from build123d import *

# Parameters (mm, degrees)
F0_W     = 4.5
F0_H     = 2.2
F1_DEPTH = 0.6
F2_W     = 4.5
F2_H     = 2.2
F3_DEPTH = 1.6
F4_R     = 1.09999
F5_R     = 0.5
F6_DEPTH = 25


# Not quite as in the source:
# - a fillet or chamfer is up to 0.001 mm smaller than in the source, because OpenCascade refuses the exact size


with BuildPart() as f1:
    # F0 (on Top) → F1 (new body)
    with BuildSketch(Plane.XY):
        with Locations((9.75, 2.6)):
            Rectangle(F0_W, F0_H)
        with BuildLine():
            Line((7.0565025569, 1.5), (7.5, 1.5))
            Line((7.5, 1.5), (7.5, 3.7))
            Line((7.5, 3.7), (7.0565025569, 3.7))
            ThreePointArc((7.0565025569, 3.7), (6.7766250144, 3.7151076306), (6.5, 3.7602549529))
            ThreePointArc((6.5, 3.7602549529), (6.2418088438, 3.8309365837), (5.9922537502, 3.9277912239))
            Line((5.9922537502, 3.9277912239), (3.6642488067, 4.9722087761))
            ThreePointArc((3.6642488067, 4.9722087761), (4.7825497586, 4.012967286), (5.2, 2.6))
            ThreePointArc((5.2, 2.6), (4.7825497586, 1.187032714), (3.6642488067, 0.2277912239))
            Line((3.6642488067, 0.2277912239), (5.9922537502, 1.2722087761))
            ThreePointArc((5.9922537502, 1.2722087761), (6.2418088438, 1.3690634163), (6.5, 1.4397450471))
            ThreePointArc((6.5, 1.4397450471), (6.7766250144, 1.4848923694), (7.0565025569, 1.5))
        make_face()
        with BuildLine():
            ThreePointArc((2.6, 0), (3.1441769851, 0.0575855159), (3.6642488067, 0.2277912239))
            ThreePointArc((3.6642488067, 0.2277912239), (4.7825497586, 1.187032714), (5.2, 2.6))
            ThreePointArc((5.2, 2.6), (4.7825497586, 4.012967286), (3.6642488067, 4.9722087761))
            ThreePointArc((3.6642488067, 4.9722087761), (3.1441769851, 5.1424144841), (2.6, 5.2))
            Line((2.6, 5.2), (2.6, 4.2))
            ThreePointArc((2.6, 4.2), (3.7313708499, 3.7313708499), (4.2, 2.6))
            ThreePointArc((4.2, 2.6), (3.7313708499, 1.4686291501), (2.6, 1))
            Line((2.6, 1), (2.6, 0))
        make_face()
        with BuildLine():
            ThreePointArc((0, 2.6), (0.7615223689, 0.7615223689), (2.6, 0))
            Line((2.6, 0), (2.6, 1))
            ThreePointArc((2.6, 1), (1, 2.6), (2.6, 4.2))
            Line((2.6, 4.2), (2.6, 5.2))
            ThreePointArc((2.6, 5.2), (0.7615223689, 4.4384776311), (0, 2.6))
        make_face()
    extrude(amount=F1_DEPTH)

    # F2 (on face) → F3 (join)
    with BuildSketch(Plane.XY.offset(0.6)):
        with Locations((9.75, 2.6)):
            Rectangle(F2_W, F2_H)
    extrude(amount=F3_DEPTH)

    # F4 (radius 1.1 in the source; OpenCascade refuses exactly that, so slightly less here)
    f4_edges = [f1.edges().sort_by_distance(p)[0] for p in [
        (9.75, 3.7, 2.2),
        (9.75, 1.5, 2.2),
    ]]
    fillet(f4_edges, radius=F4_R)

    # F5 (on face) → F6 (cut)
    with BuildSketch(Plane.YZ.offset(12)):
        with Locations((2.6, 1.1)):
            Circle(F5_R)
    extrude(amount=-F6_DEPTH, mode=Mode.SUBTRACT)


solid = f1.part
Verification items for the finished model (mm, model axes). A direction names the side the tool comes from. Coordinates: 2 decimals unless noted, no trailing zeros. Loops run counter-clockwise (first coordinate to the right, second up) from the corner with the lowest first, then second, coordinate; pieces in that order, holes last. Notation, with made-up numbers: (78.25, -19) -> (83.25, -19) arc R24 ccw to (83.25, 8) -> close; hole circle Ø11 at (14.5, 83.25). An arc over 180 degrees is marked (long way). Answer as CSV lines item,"result".
1) Cross-section at A-A, the plane z = 0.35. Record the cut outline in (x, y), then the cut area to 3 significant figures.
Found:
outline,"(3.66, 0.23) -> (5.99, 1.27) arc R2.6 cw to (7.06, 1.5) -> (12, 1.5) -> (12, 3.7) -> (7.06, 3.7) arc R2.6 cw to (5.99, 3.93) -> (3.66, 4.97) arc R2.6 ccw (long way) to start; hole circle Ø3.2 at (2.6, 2.6)"
area,"29.9 mm2"
2) Thickness scan on L1, parallel to Y at x = 9.6, z = 1.1; L2, parallel to Z at x = 9.25, y = 2.6; L3, parallel to X at y = 3.25, z = 0.8. Record the ranges inside material, lowest first. Write a range as from..to.
Found:
L1,"y = 1.5..2.1, 3.1..3.7"
L2,"z = 0..0.6, 1.6..2.2"
L3,"x = 7.5..12"
3) Release check for a two-part mould opening along Z. For faces 4 (the cylindrical face through (9.782, 3.369, 1.886)), 5 (the flat face through (9.5, 1.5, 0.5)), 6 (the flat face through (6, 3, 0)), 7 (the cylindrical face through (9.8, 2.9, 1.5)) record: +Z half, -Z half, draft (parallel to the pull), parting line (faces both ways), or undercut.
Found:
face 4,"+Z half"
face 5,"draft"
face 6,"-Z half"
face 7,"undercut"
4) Tool access check on faces 1 (the flat face through (7.5, 2.3, 1.7)), 2 (the flat face through (9.5, 3.7, 0.5)), 3 (the cylindrical face through (9.782, 1.831, 1.886)). Record the directions out of +Z, -Z, +X, -X, +Y, -Y that give a thin tool (end or side, any length) a straight path to the whole face; none if there is none.
Found:
face 1,"+Z, -X, +Y, -Y"
face 2,"+Z, -Z, +X, +Y"
face 3,"+Z, +X, -X, -Y"
5) Cross-section at C-C, the plane y = 3.55. Record the cut outline in (x, z).
Found:
outline,"(0.18, 0) -> (1.31, 0) -> (1.31, 0.6) -> (0.18, 0.6) -> close; (3.89, 0) -> (12, 0) -> (12, 1.65) -> (7.5, 1.65) -> (7.5, 0.6) -> (3.89, 0.6) -> close"
6) Depth check by flat-ended pin: pin 1 (0.8 mm diameter, centred on y = 3, z = 1.5, fed in from -X); pin 2 (1 mm diameter, centred on y = 2.5, z = 1, fed in from +X); pin 3 (0.9 mm diameter, centred on x = 8.5, z = 1, fed in from -Y); pin 4 (2 mm diameter, centred on x = 8, y = 4, fed in from +Z). Enter the tip coordinate at first touch or a pass-through.
Found:
pin 1,"stops at x = 7.5"
pin 2,"stops at x = 12"
pin 3,"stops at y = 1.5"
pin 4,"stops at z = 2.12"
7) Cross-section at B-B, the plane x = 2.75. Record the cut outline in (y, z), then the cut area to 3 significant figures.
Found:
outline,"(0, 0) -> (1.01, 0) -> (1.01, 0.6) -> (0, 0.6) -> close; (4.19, 0) -> (5.2, 0) -> (5.2, 0.6) -> (4.19, 0.6) -> close"
area,"1.20 mm2"
8) Cross-section at D-D, the plane z = 0.85. Record the cut outline in (x, y), then the cut area to 3 significant figures.
Found:
outline,"(7.5, 1.5) -> (12, 1.5) -> (12, 2.17) -> (7.5, 2.17) -> close; (7.5, 3.03) -> (12, 3.03) -> (12, 3.7) -> (7.5, 3.7) -> close"
area,"6.00 mm2"
